from build123d import *


with BuildPart() as part:
    # Эскиз4 → Повернуть1 (revolve)
    with BuildSketch(Plane.XY, mode=Mode.PRIVATE) as revolve_1_sk:
        Polygon((-30, 30), (-30, 25.082903769), (-28, 23.082903769), (-14, 15), (-14, 3), (-8, 3), (-8, 13), (0, 13), (0, 30), align=None)
    revolve(revolve_1_sk.sketch.rotate(Axis((-30, 0, 0), (1, 0, 0)), 90), axis=Axis((-30, 0, 0), (1, 0, 0)))


solid = part.part
The model under review builds one solid part; all positions refer to its coordinate system, in mm. A direction names the side the tool comes from. Give positions to 0.01 mm unless a question says otherwise; leave off trailing zeros. Loops run counter-clockwise (first coordinate to the right, second up) from the corner with the lowest first, then second, coordinate; pieces in that order, holes last. Notation, with made-up numbers: (62.5, 87) -> (105.5, 87) arc R18 ccw to (105.5, 112) -> close; hole circle Ø7 at (83, 47.5). An arc over 180 degrees is marked (long way). Write each question's results on one line, items separated by ' | '.
1) Take a section at D-D, the plane x = -17.75. Give the boundary of the cut face in (y, z).
Conclusion:
outline: circle Ø60 at (0, 0); hole circle Ø34.33 at (0, 0)
2) Take a section at C-C, the plane x = -10. Give the boundary of the cut face in (y, z).
Conclusion:
outline: circle Ø60 at (0, 0); hole circle Ø6 at (0, 0)
3) Tool access review of faces 1 (the face through (0, 6, -13)), 2 (the face through (-14, -4, 0)), 3 (the face through (-3.944, 7.91, -10.316)): name each direction out of +Z, -Z, +X, -X, +Y, -Y from which nothing blocks a thin tool from reaching the whole face with its end or side.
Conclusion:
face 1: +Z, -Z, +X, +Y, -Y | face 2: -X | face 3: +X
4) Draft analysis for pull direction Y (two halves, no side actions). For faces 4 (the face through (-14.7, -4.6, 14.7)), 5 (the face through (-30, 24.3, -6.8)), 6 (the face through (-15.21, -25.296, 16.128)), state which applies: pulls with the +Y half, pulls with the -Y half, needs draft (parallel to the pull), parting line crosses it, or undercut.
Conclusion:
face 4: undercut | face 5: needs draft | face 6: parting line crosses it
5) For line 1 along Y through (x, z) = (-4.25, 0); line 2 along Z through (x, y) = (-25, -0.5) (3 decimals); line 3 along Z through (x, y) = (-24.5, 13), list the stretches that pass through material, from the lowest coordinate up. Write a range as from..to.
Conclusion:
line 1: y = -30..-13, 13..30 | line 2: z = -29.996..-21.345, 21.345..29.996 | line 3: z = -27.04..-16.57, 16.57..27.04
6) Insertion check: pin 1 Ø8 at (y, z) = (-3, 2.5) entering from +X; pin 2 Ø3 at (x, z) = (-4, -6) entering from -Y; pin 3 Ø9 at (y, z) = (-2, -1.5) entering from -X. Each pin has a flat end and moves straight along its axis. Give the tip position at first contact, or say it passes through.
Conclusion:
pin 1: stops at x = -8 | pin 2: stops at y = -29.66 | pin 3: stops at x = -14
7) Take a section at A-A, the plane z = 0. Give the boundary of the cut face in (x, y), plus the area to 3 significant figures.
Conclusion:
outline: (-30, -30) -> (0, -30) -> (0, -13) -> (-8, -13) -> (-8, -3) -> (-14, -3) -> (-14, -15) -> (-28, -23.08) -> (-30, -25.08) -> close; (-30, 25.08) -> (-28, 23.08) -> (-14, 15) -> (-14, 3) -> (-8, 3) -> (-8, 13) -> (0, 13) -> (0, 30) -> (-30, 30) -> close | area: 927 mm^2
